Autodesk Inventor part; units mm, degrees
ref_plane "YZ Plane" through (0, 0, 0) normal (1, 0, 0) x (0, 1, 0)
ref_plane "XZ Plane" through (0, 0, 0) normal (0, 1, 0) x (-1, 0, 0)
ref_plane "XY Plane" through (0, 0, 0) normal (0, 0, 1) x (1, 0, 0)
sketch "Sketch1" plane through (0, 0, 0) normal (1, 0, 0) x (0, 1, 0)
  point P0 (0, 0)
sketch "Sketch2" plane through (0, 0, 0) normal (1, 0, 0) x (0, 1, 0)
  circle A0 centre (0, 0) radius 31.5
  arc A1 (40, 69.282) -> (-40, 69.282) centre (0, 0) ccw
  line L0 (0, 0) -> (-40, 69.282) construction
  line L1 (0, 0) -> (80, 0) construction
  line L2 (0, 0) -> (40, 69.282) construction
  line L3 (40, 69.282) -> (45, 77.9423)
  line L4 (-40, 69.282) -> (-45, 77.9423)
  arc A2 (40, 69.282) -> (45, 77.9423) centre (42.5, 73.6122) ccw
  arc A3 (-45, 77.9423) -> (-40, 69.282) centre (-42.5, 73.6122) ccw
  arc A4 (-40, -69.282) -> (40, -69.282) centre (0, 0) ccw
  line L5 (0, 0) -> (40, -69.282) construction
  line L6 (0, 0) -> (80, 0) construction
  line L7 (0, 0) -> (-40, -69.282) construction
  line L8 (-40, -69.282) -> (-45, -77.9423)
  arc A5 (45, -77.9423) -> (40, -69.282) centre (42.5, -73.6122) ccw
  arc A6 (-40, -69.282) -> (-45, -77.9423) centre (-42.5, -73.6122) ccw
  arc A7 (45, 77.9423) -> (-45, 77.9423) centre (0, 0) ccw
  arc A8 (-45, -77.9423) -> (45, -77.9423) centre (0, 0) ccw
  arc A9 (40, 69.282) -> (-40, 69.282) centre (0, 0) ccw
  arc A10 (-40, -69.282) -> (40, -69.282) centre (0, 0) ccw
  line L9 (0, 0) -> (-72.5, 0)
  line L10 (-72.5, 0) -> (-72.5, -15.5)
  line L11 (-72.5, -15.5) -> (-72.5, -35.5)
  line L12 (-72.5, -35.5) -> (-72.5, -51)
  line L13 (-121.003, -51) -> (-188, -51)
  line L14 (-188, -51) -> (-188, -35.5)
  line L15 (-188, -35.5) -> (-72.5, -35.5)
  line L16 (-72.5, -15.5) -> (-188, -15.5)
  line L17 (-188, -15.5) -> (-188, -35.5)
  circle A11 centre (-72.5, -25.5) radius 10
  circle A12 centre (-188, -25.5) radius 10
  line L18 (-72.5, 0) -> (-72.5, 15.5)
  line L19 (-72.5, 15.5) -> (-72.5, 35.5)
  line L20 (-72.5, 35.5) -> (-72.5, 51)
  line L21 (-112.428, 51) -> (-188, 51)
  line L22 (-188, 51) -> (-188, 35.5)
  line L23 (-188, 35.5) -> (-72.5, 35.5)
  line L24 (-72.5, 15.5) -> (-188, 15.5)
  line L25 (-188, 15.5) -> (-188, 35.5)
  circle A13 centre (-188, 25.5) radius 10
  circle A14 centre (-72.5, 25.5) radius 10
  line L26 (-188, 51) -> (-188, 51)
  line L27 (-208, 31) -> (-208, -31)
  line L28 (-188, -51) -> (-188, -51)
  arc A15 (-208, -31) -> (-188, -51) centre (-188, -31) ccw
  arc A16 (-188, 51) -> (-208, 31) centre (-188, 31) ccw
  line L29 (-188, 25.5) -> (-72.5, 25.5)
  arc A17 (-98.8167, 35.5) -> (-103.8497, 15.5) centre (0, 0) ccw
  arc A18 (-71.5049, -71.5031) -> (-121.003, -51) centre (-121.003, -121) ccw
  arc A19 (-112.428, 51) -> (-68.365, 66.6083) centre (-112.428, 121) ccw
  line L30 (0, 0) -> (62.5, 0)
  line L31 (62.5, 0) -> (62.5, 62.3398)
  line L32 (62.5, 0) -> (62.5, -69.098)
  arc A20 (-71.5049, -71.5031) -> (52.978, -86.1335) centre (0, 0) ccw
  arc A21 (53.7659, 78.8649) -> (-68.365, 66.6083) centre (0, 0) ccw
  arc A22 (62.5, 62.3398) -> (53.7659, 78.8649) centre (42.5, 62.3398) ccw
  arc A23 (52.978, -86.1335) -> (62.5, -69.098) centre (42.5, -69.098) ccw
  point P0 (-208, 51)
  point P1 (-87.3193, 51)
  point P2 (-87.3193, -51)
  point P3 (62.5, 72.1401)
  point P4 (62.5, -79.4947)
  dimension "d0" = 63
  dimension "d4" = 120
  dimension "d5" = 60
  dimension "d6" = 60
  dimension "d7" = 60
  dimension "d8" = 10
  dimension "d9" = 10
  dimension "d10" = 72.5
  dimension "d11" = 15.5
  dimension "d12" = 20
  dimension "d13" = 15.5
  dimension "d14" = 115.5
  dimension "d15" = 15.5
  dimension "d16" = 20
  dimension "d17" = 15.5
  dimension "d18" = 20
  dimension "d20" = 20
  dimension "d21" = 20
  dimension "d22" = 115.5
  dimension "d23" = 70
  dimension "d24" = 70
  dimension "d25" = 62.5
  dimension "d26" = 20
  dimension "d27" = 20
extrude "Extrusion1" add sketch "Sketch2" along normal blind 20 contours L30 L32 A23 A20 A18 L13 L14 L15 A11 L10 L9 A0 | A0 L9 L18 A14 L23 L22 L21 A19 A21 A22 L31 L30 | L10 L16 A12 L14 A15 L27 A16 L22 A13 L24 L18
Geometry: final body of the model. Coordinates: model frame, mm. A direction names the side the tool comes from. Give positions to 0.01 mm unless a question says otherwise; leave off trailing zeros. Loops run counter-clockwise (first coordinate to the right, second up) from the corner with the lowest first, then second, coordinate; pieces in that order, holes last. Notation, with made-up numbers: (6.25, 30.25) -> (49.25, 30.25) arc R26 ccw to (49.25, 49.25) -> close; hole circle Ø5 at (72, 45). An arc over 180 degrees is marked (long way). Return JSON: item names as keys, results as strings.
Item 1: Section C-C, the plane z = 25.5. Output: boundary loops of the cut face in (x, y).
Filled in:
{"outline": "(0, -208) -> (20, -208) -> (20, -198) -> (0, -198) -> close; (0, -62.5) -> (20, -62.5) -> (20, -18.49) -> (0, -18.49) -> close; (0, 18.49) -> (20, 18.49) -> (20, 62.5) -> (0, 62.5) -> close"}
Item 2: Section D-D, the plane y = -104.5. Output: boundary loops of the cut face in (x, z).
Filled in:
{"outline": "(0, -52.97) -> (20, -52.97) -> (20, -35.5) -> (0, -35.5) -> close; (0, -15.5) -> (20, -15.5) -> (20, 15.5) -> (0, 15.5) -> close; (0, 35.5) -> (20, 35.5) -> (20, 51.45) -> (0, 51.45) -> close"}
Item 3: Section A-A, the plane x = 4. Count the separate pieces of the cut face and the enclosed holes in it, plus the area to 3 significant figures.
Filled in:
{"separate pieces": "1", "enclosed holes": "5", "area": "28,000 mm^2"}
Item 4: Section B-B, the plane y = 0. Output: boundary loops of the cut face in (x, z), plus the area to 3 significant figures.
Filled in:
{"outline": "(0, -101.12) -> (20, -101.12) -> (20, -90) -> (0, -90) -> close; (0, -80) -> (20, -80) -> (20, -31.5) -> (0, -31.5) -> close; (0, 31.5) -> (20, 31.5) -> (20, 80) -> (0, 80) -> close; (0, 90) -> (20, 90) -> (20, 95.45) -> (0, 95.45) -> close", "area": "2,270 mm^2"}
Item 5: Line query: line 1 (Z direction, x = 10.25, y = 0); line 2 (Z direction, x = 6, y = -150); line 3 (Y direction, x = 11.5, z = 0). Output: solid intervals per line, ascending.
Filled in:
{"line 1": "-101.12 to -90, -80 to -31.5, 31.5 to 80, 90 to 95.45", "line 2": "-51 to -35.5, -15.5 to 15.5, 35.5 to 51", "line 3": "-208 to -31.5, 31.5 to 62.5"}
Item 6: Pin query (flat end, axial travel): P1, Ø6, axis at x = 7, y = -103, coming from the +Z side; P2, Ø12, axis at y = -57, z = 2, coming from the -X side; P3, Ø10, axis at x = 3, z = -75.5, coming from the +Y side; P4, Ø1, axis at x = 6, y = -32, coming from the -Z side. Return the tip coordinate at first contact, or that it passes through.
Filled in:
{"P1": "z = 52.11", "P2": "x = 0", "P3": "y = 62.45", "P4": "z = -96.09"}
Item 7: Access query for faces 1 (the flat face through (10, -131, 35.5)), 2 (the flat face through (10, -150, 51)), 3 (the flat face through (10, 62.5, -2)). Directions: +Z, -Z, +X, -X, +Y, -Y. A direction counts if a zero-diameter tool reaches every point of the face in a straight line with its end or side. Return the directions, or none.
Filled in:
{"face 1": "+X, -X", "face 2": "+Z, +X, -X, -Y", "face 3": "+Z, -Z, +X, -X, +Y"}
